Geometry check sheet. Reference: drawing and pictorial views, mm from the part's lowest x, y, z. A direction names the side the tool comes from. Round coordinates to 2 decimals unless told otherwise and drop trailing zeros. Write each loop counter-clockwise with the first axis right and the second up, starting at its lowest first coordinate (ties: lowest second). Pieces come first, ordered by that corner, then holes.
Item 1: Section check C-C, the plane x = 5.75. Record the cut outline in (y, z) (1 decimal).
Item 2: Section check D-D, the plane z = 4.75. Record the cut outline in (x, y), plus the area to 3 significant figures.
Item 3: Release check for a two-part mould opening along Z. For the marked faces 1, 2 and 3 record: pulls with the +Z half, pulls with the -Z half, needs draft (parallel to the pull), parting line crosses it, or undercut.
Item 4: Material ranges on line 1 along Z through (x, y) = (13.75, 10.25) (1 decimal); line 2 along Y through (x, z) = (4.75, 11.5); line 3 along X through (y, z) = (5, 13.75) (1 decimal), recorded low to high.
Item 5: Set-up check for the marked faces 4, 5, 6, 7 and 8: record each of +Z, -Z, +X, -X, +Y, -Y from which the full face is reachable in a straight line by a thin tool's end or side.
Item 6: Section check B-B, the plane z = 2. State how many separate pieces and enclosed holes the cut face has.
Item 7: Depth check by flat-ended pin: pin 1 (1.3 mm diameter, centred on y = 8.5, z = 3, fed in from +X); pin 2 (0.7 mm diameter, centred on x = 4.25, z = 1.82, fed in from -Y); pin 3 (1 mm diameter, centred on x = 10.5, y = 8, fed in from -Z) (1 decimal); pin 4 (1.3 mm diameter, centred on y = 11, z = 2, fed in from -X). Enter the tip coordinate at first touch or a pass-through.
Item 8: Section check A-A, the plane y = 13.25. Record the cut outline in (x, z) (1 decimal).
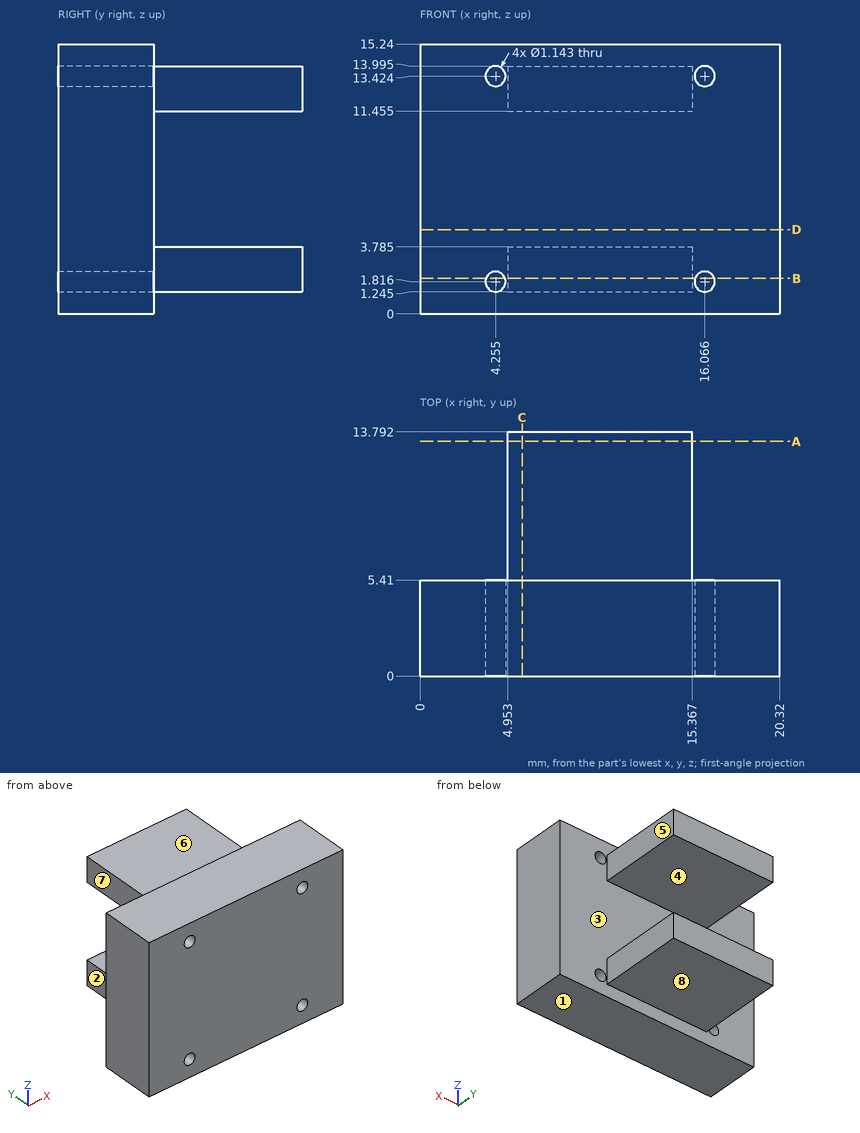
Values found:
1. outline: (0, 0) - (5.4, 0) - (5.4, 1.2) - (13.8, 1.2) - (13.8, 3.8) - (5.4, 3.8) - (5.4, 11.5) - (13.8, 11.5) - (13.8, 14) - (5.4, 14) - (5.4, 15.2) - (0, 15.2) - close
2. outline: (0, 0) - (20.32, 0) - (20.32, 5.41) - (0, 5.41) - close
2. area: 110 mm2
3. face 1: pulls with the -Z half
3. face 2: needs draft
3. face 3: undercut
4. line 1: z = 1.2 to 3.8, 11.5 to 14
4. line 2: y = 0 to 5.41
4. line 3: x = 0 to 3.8, 4.7 to 15.6, 16.5 to 20.3
5. face 4: +X, -X, +Y
5. face 5: +Z, -Z, +X, +Y
5. face 6: +Z, +X, -X, +Y
5. face 7: +Z, -Z, -X, +Y
5. face 8: -Z, +X, -X, +Y
6. separate pieces: 3
6. enclosed holes: 0
7. pin 1: stops at x = 15.37
7. pin 2: passes through
7. pin 3: stops at z = 1.2
7. pin 4: stops at x = 4.95
8. outline: (5, 1.2) - (15.4, 1.2) - (15.4, 3.8) - (5, 3.8) - close; (5, 11.5) - (15.4, 11.5) - (15.4, 14) - (5, 14) - close
